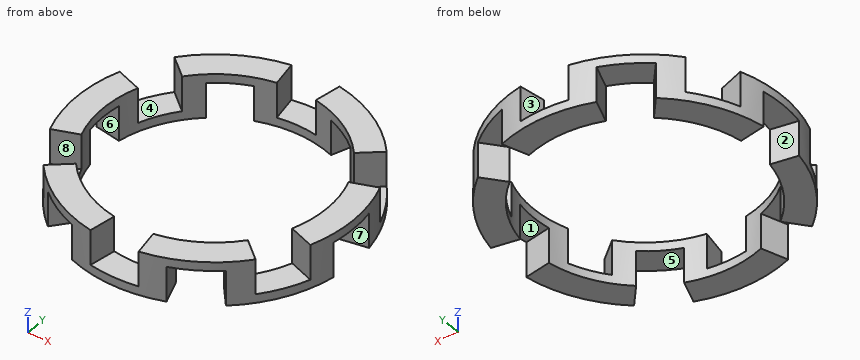
```python
from build123d import *

# Parameters (mm, degrees)
F0_R     = 31.5
F0_R_2   = 25.5
F1_DEPTH = 5
F5_DEPTH = 25
F7_DEPTH = 25
F8_DEPTH = 4.25
F9_DEPTH = 4.25


with BuildPart() as f1:
    # F0 (on Top) → F1 (new body, symmetric)
    with BuildSketch(Plane.XY):
        Circle(F0_R)
        Circle(F0_R_2, mode=Mode.SUBTRACT)
    extrude(amount=F1_DEPTH, both=True)

    # F4 (on offset) → F5 (cut)
    with BuildSketch(Plane.XY.offset(1.25)):
        with BuildLine():
            ThreePointArc((19.5341332995, 16.391084047), (22.0836477965, 12.75), (23.96216183, 8.7215136548))
            Line((23.96216183, 8.7215136548), (29.6003175548, 10.7736345148))
            ThreePointArc((29.6003175548, 10.7736345148), (27.2798002192, 15.75), (24.1303999582, 20.2478097051))
            Line((24.1303999582, 20.2478097051), (19.5341332995, 16.391084047))
        make_face()
        with BuildLine():
            Line((-5.4699175965, 31.0214442199), (-4.4280285305, 25.1125977018))
            ThreePointArc((-4.4280285305, 25.1125977018), (0, 25.5), (4.4280285305, 25.1125977018))
            Line((4.4280285305, 25.1125977018), (5.4699175965, 31.0214442199))
            ThreePointArc((5.4699175965, 31.0214442199), (0, 31.5), (-5.4699175965, 31.0214442199))
        make_face()
        with BuildLine():
            Line((-29.6003175548, 10.7736345148), (-23.96216183, 8.7215136548))
            ThreePointArc((-23.96216183, 8.7215136548), (-22.0836477965, 12.75), (-19.5341332995, 16.391084047))
            Line((-19.5341332995, 16.391084047), (-24.1303999582, 20.2478097051))
            ThreePointArc((-24.1303999582, 20.2478097051), (-27.2798002192, 15.75), (-29.6003175548, 10.7736345148))
        make_face()
        with BuildLine():
            Line((-24.1303999582, -20.2478097051), (-19.5341332995, -16.391084047))
            ThreePointArc((-19.5341332995, -16.391084047), (-22.0836477965, -12.75), (-23.96216183, -8.7215136548))
            Line((-23.96216183, -8.7215136548), (-29.6003175548, -10.7736345148))
            ThreePointArc((-29.6003175548, -10.7736345148), (-27.2798002192, -15.75), (-24.1303999582, -20.2478097051))
        make_face()
        with BuildLine():
            Line((5.4699175965, -31.0214442199), (4.4280285305, -25.1125977018))
            ThreePointArc((4.4280285305, -25.1125977018), (0, -25.5), (-4.4280285305, -25.1125977018))
            Line((-4.4280285305, -25.1125977018), (-5.4699175965, -31.0214442199))
            ThreePointArc((-5.4699175965, -31.0214442199), (0, -31.5), (5.4699175965, -31.0214442199))
        make_face()
        with BuildLine():
            Line((29.6003175548, -10.7736345148), (23.96216183, -8.7215136548))
            ThreePointArc((23.96216183, -8.7215136548), (22.0836477965, -12.75), (19.5341332995, -16.391084047))
            Line((19.5341332995, -16.391084047), (24.1303999582, -20.2478097051))
            ThreePointArc((24.1303999582, -20.2478097051), (27.2798002192, -15.75), (29.6003175548, -10.7736345148))
        make_face()
    extrude(amount=F5_DEPTH, mode=Mode.SUBTRACT)

    # F6 (on offset) → F7 (cut)
    with BuildSketch(Plane.XY.offset(-1.25)):
        with BuildLine():
            Line((10.7736345148, 29.6003175548), (8.7215136548, 23.96216183))
            ThreePointArc((8.7215136548, 23.96216183), (12.75, 22.0836477965), (16.391084047, 19.5341332995))
            Line((16.391084047, 19.5341332995), (20.2478097051, 24.1303999582))
            ThreePointArc((20.2478097051, 24.1303999582), (15.75, 27.2798002192), (10.7736345148, 29.6003175548))
        make_face()
        with BuildLine():
            Line((-8.7215136548, 23.96216183), (-10.7736345148, 29.6003175548))
            ThreePointArc((-10.7736345148, 29.6003175548), (-15.75, 27.2798002192), (-20.2478097051, 24.1303999582))
            Line((-20.2478097051, 24.1303999582), (-16.391084047, 19.5341332995))
            ThreePointArc((-16.391084047, 19.5341332995), (-12.75, 22.0836477965), (-8.7215136548, 23.96216183))
        make_face()
        with BuildLine():
            Line((-25.1125977018, 4.4280285305), (-31.0214442199, 5.4699175965))
            ThreePointArc((-31.0214442199, 5.4699175965), (-31.5, 0), (-31.0214442199, -5.4699175965))
            Line((-31.0214442199, -5.4699175965), (-25.1125977018, -4.4280285305))
            ThreePointArc((-25.1125977018, -4.4280285305), (-25.5, 0), (-25.1125977018, 4.4280285305))
        make_face()
        with BuildLine():
            Line((-16.391084047, -19.5341332995), (-20.2478097051, -24.1303999582))
            ThreePointArc((-20.2478097051, -24.1303999582), (-15.75, -27.2798002192), (-10.7736345148, -29.6003175548))
            Line((-10.7736345148, -29.6003175548), (-8.7215136548, -23.96216183))
            ThreePointArc((-8.7215136548, -23.96216183), (-12.75, -22.0836477965), (-16.391084047, -19.5341332995))
        make_face()
        with BuildLine():
            Line((8.7215136548, -23.96216183), (10.7736345148, -29.6003175548))
            ThreePointArc((10.7736345148, -29.6003175548), (15.75, -27.2798002192), (20.2478097051, -24.1303999582))
            Line((20.2478097051, -24.1303999582), (16.391084047, -19.5341332995))
            ThreePointArc((16.391084047, -19.5341332995), (12.75, -22.0836477965), (8.7215136548, -23.96216183))
        make_face()
        with BuildLine():
            Line((25.1125977018, -4.4280285305), (31.0214442199, -5.4699175965))
            ThreePointArc((31.0214442199, -5.4699175965), (31.5, 0), (31.0214442199, 5.4699175965))
            Line((31.0214442199, 5.4699175965), (25.1125977018, 4.4280285305))
            ThreePointArc((25.1125977018, 4.4280285305), (25.5, 0), (25.1125977018, -4.4280285305))
        make_face()
    extrude(amount=-F7_DEPTH, mode=Mode.SUBTRACT)

    # F8 (cut): faces of the model
    f8_faces = [f1.faces().sort_by_distance(p)[0] for p in [
        (-24.6473051281, -14.2301282505, 1.25),
        (-24.6473051281, 14.2301282505, 1.25),
        (0, 28.460256501, 1.25),
        (24.6473051281, 14.2301282505, 1.25),
        (24.6473051281, -14.2301282505, 1.25),
        (0, -28.460256501, 1.25),
    ]]
    extrude(f8_faces, amount=-F8_DEPTH, mode=Mode.SUBTRACT)

    # F9 (cut): faces of the model
    f9_faces = [f1.faces().sort_by_distance(p)[0] for p in [
        (-14.2301282505, -24.6473051281, -1.25),
        (14.2301282505, -24.6473051281, -1.25),
        (28.460256501, 0, -1.25),
        (14.2301282505, 24.6473051281, -1.25),
        (-14.2301282505, 24.6473051281, -1.25),
        (-28.460256501, 0, -1.25),
    ]]
    extrude(f9_faces, amount=-F9_DEPTH, mode=Mode.SUBTRACT)


solid = f1.part
```
Input: part model. Units: mm. Frame: model coordinates. Face numbers are marked on the shaded views. A direction names the side the tool comes from. Coordinates: 2 decimals unless noted, no trailing zeros. Loops run counter-clockwise (first coordinate to the right, second up) from the corner with the lowest first, then second, coordinate; pieces in that order, holes last.
Q1. Section D-D, the plane x = 28.5. Return the cut outline in (y, z), and give its area (3 significant figures).
Results are:
outline: (-13.42, -5) - (-5.03, -5) - (-5.03, 3) - (5.03, 3) - (5.03, -5) - (13.42, -5) - (13.42, -3) - (10.37, -3) - (10.37, 5) - (-10.37, 5) - (-10.37, -3) - (-13.42, -3) - close
area: 139 mm2
Q2. Line query: line 1 along X through (y, z) = (0, 3.25); line 2 along X through (y, z) = (27, -1). Output: solid intervals per line, ascending.
Results are:
line 1: x = -31.5 to -25.5, 25.5 to 31.5
line 2: x = -9.83 to -4.76, 4.76 to 9.83
Q3. Section A-A, the plane y = 0. Return the cut outline in (x, z).
Results are:
outline: (-31.5, 3) - (-25.5, 3) - (-25.5, 5) - (-31.5, 5) - close; (25.5, 3) - (31.5, 3) - (31.5, 5) - (25.5, 5) - close
Q4. Section B-B, the plane x = 0. Return the cut outline in (y, z), and give its area (3 significant figures).
Results are:
outline: (-31.5, -5) - (-25.5, -5) - (-25.5, -3) - (-31.5, -3) - close; (25.5, -5) - (31.5, -5) - (31.5, -3) - (25.5, -3) - close
area: 24.0 mm2
Q5. Mould query, pull axis X, two halves, no side actions, for the marked faces 6, 7 and 8. Classes: +X half, -X half, draft (parallel to the pull), parting line (faces both ways), or undercut.
Results are:
face 6: -X half
face 7: +X half
face 8: undercut
Q6. Contact query for flat-ended pins moving along their axis: pin 1 (11 mm diameter, centred on x = 24.5, y = -15, fed in from +Z); pin 2 (1.5 mm diameter, centred on x = -9.5, z = -0.5, fed in from +Y); pin 3 (8 mm diameter, centred on x = 26.5, y = 14.5, fed in from +Z); pin 4 (5 mm diameter, centred on x = -3, z = 1.5, fed in from -Y). Output: stop coordinate, or through.
Results are:
pin 1: stops at z = 5
pin 2: stops at y = 30.26
pin 3: stops at z = -3
pin 4: stops at y = -31.02
Q7. Section C-C, the plane z = 1. Give the number of separate pieces and of enclosed holes in the cut face, and give its area (3 significant figures).
Results are:
separate pieces: 12
enclosed holes: 0
area: 358 mm2
Q8. Set-up query: the marked faces 1, 2, 3, 4 and 5. Return all of +Z, -Z, +X, -X, +Y, -Y with unobstructed straight access to the full face (end or side cutting, diameter ignored); none if empty.
Results are:
face 1: -Z, +X
face 2: -Z, -X
face 3: +Z, +Y
face 4: +Z
face 5: -Z
